```python
from build123d import *

# Parameters (mm, degrees)
SALIENTE_EXTRUIR1_DEPTH = 15
CROQUIS2_R              = 7
CORTAR_EXTRUIR1_DEPTH   = 135.246042772


with BuildPart() as part:
    # Croquis1 → Saliente-Extruir1 (new body)
    with BuildSketch(Plane.XY):
        with BuildLine():
            ThreePointArc((22.960111456, -43.287795993), (49, 0), (22.960111456, 43.287795993))
            ThreePointArc((22.960111456, 43.287795993), (17.471680778, 49.356927241), (17.149797537, 57.533333333))
            ThreePointArc((17.149797537, 57.533333333), (12.479188654, 75.97188693), (-6.126315717, 79.925373134))
            ThreePointArc((-6.126315717, 79.925373134), (-35.730309716, 61.63434209), (-55.523644659, 33.012983471))
            ThreePointArc((-55.523644659, 33.012983471), (-64.981782963, 22.905981014), (-78.737580645, 21.361342246))
            ThreePointArc((-78.737580645, 21.361342246), (-106, 0), (-78.737580645, -21.361342246))
            ThreePointArc((-78.737580645, -21.361342246), (-64.981782963, -22.905981014), (-55.523644659, -33.012983471))
            ThreePointArc((-55.523644659, -33.012983471), (-35.730309716, -61.63434209), (-6.126315717, -79.925373134))
            ThreePointArc((-6.126315717, -79.925373134), (12.479188654, -75.97188693), (17.149797537, -57.533333333))
            ThreePointArc((17.149797537, -57.533333333), (17.471680778, -49.356927241), (22.960111456, -43.287795993))
        make_face()
    extrude(amount=-SALIENTE_EXTRUIR1_DEPTH)

    # Croquis2 → Cortar-Extruir1 (cut, through all)
    with BuildSketch(Plane.XY):
        with Locations((0, 63)):
            Circle(CROQUIS2_R)
        with Locations((-84, 0)):
            Circle(CROQUIS2_R)
        with Locations((0, -63)):
            Circle(CROQUIS2_R)
        with BuildLine():
            Line((-2, 30.535898385), (-2, 26.925824036))
            ThreePointArc((-2, 26.925824036), (-6.988114218, 26.07999731), (-11.73086121, 24.318447633))
            Line((-11.73086121, 24.318447633), (-13.535898385, 27.444863729))
            ThreePointArc((-13.535898385, 27.444863729), (-19, 32.908965344), (-17, 25.444863729))
            Line((-17, 25.444863729), (-15.194962825, 22.318447633))
            ThreePointArc((-15.194962825, 22.318447633), (-19.091883092, 19.091883092), (-22.318447633, 15.194962825))
            Line((-22.318447633, 15.194962825), (-25.444863729, 17))
            ThreePointArc((-25.444863729, 17), (-32.908965344, 19), (-27.444863729, 13.535898385))
            Line((-27.444863729, 13.535898385), (-24.318447633, 11.73086121))
            ThreePointArc((-24.318447633, 11.73086121), (-26.07999731, 6.988114218), (-26.925824036, 2))
            Line((-26.925824036, 2), (-30.535898385, 2))
            ThreePointArc((-30.535898385, 2), (-38, 0), (-30.535898385, -2))
            Line((-30.535898385, -2), (-26.925824036, -2))
            ThreePointArc((-26.925824036, -2), (-26.07999731, -6.988114218), (-24.318447633, -11.73086121))
            Line((-24.318447633, -11.73086121), (-27.444863729, -13.535898385))
            ThreePointArc((-27.444863729, -13.535898385), (-32.908965344, -19), (-25.444863729, -17))
            Line((-25.444863729, -17), (-22.318447633, -15.194962825))
            ThreePointArc((-22.318447633, -15.194962825), (-19.091883092, -19.091883092), (-15.194962825, -22.318447633))
            Line((-15.194962825, -22.318447633), (-17, -25.444863729))
            ThreePointArc((-17, -25.444863729), (-19, -32.908965344), (-13.535898385, -27.444863729))
            Line((-13.535898385, -27.444863729), (-11.73086121, -24.318447633))
            ThreePointArc((-11.73086121, -24.318447633), (-6.988114218, -26.07999731), (-2, -26.925824036))
            Line((-2, -26.925824036), (-2, -30.535898385))
            ThreePointArc((-2, -30.535898385), (0, -38), (2, -30.535898385))
            Line((2, -30.535898385), (2, -26.925824036))
            ThreePointArc((2, -26.925824036), (6.988114218, -26.07999731), (11.73086121, -24.318447633))
            Line((11.73086121, -24.318447633), (13.535898385, -27.444863729))
            ThreePointArc((13.535898385, -27.444863729), (19, -32.908965344), (17, -25.444863729))
            Line((17, -25.444863729), (15.194962825, -22.318447633))
            ThreePointArc((15.194962825, -22.318447633), (19.091883092, -19.091883092), (22.318447633, -15.194962825))
            Line((22.318447633, -15.194962825), (25.444863729, -17))
            ThreePointArc((25.444863729, -17), (32.908965344, -19), (27.444863729, -13.535898385))
            Line((27.444863729, -13.535898385), (24.318447633, -11.73086121))
            ThreePointArc((24.318447633, -11.73086121), (26.07999731, -6.988114218), (26.925824036, -2))
            Line((26.925824036, -2), (30.535898385, -2))
            ThreePointArc((30.535898385, -2), (38, 0), (30.535898385, 2))
            Line((30.535898385, 2), (26.925824036, 2))
            ThreePointArc((26.925824036, 2), (26.07999731, 6.988114218), (24.318447633, 11.73086121))
            Line((24.318447633, 11.73086121), (27.444863729, 13.535898385))
            ThreePointArc((27.444863729, 13.535898385), (32.908965344, 19), (25.444863729, 17))
            Line((25.444863729, 17), (22.318447633, 15.194962825))
            ThreePointArc((22.318447633, 15.194962825), (19.091883092, 19.091883092), (15.194962825, 22.318447633))
            Line((15.194962825, 22.318447633), (17, 25.444863729))
            ThreePointArc((17, 25.444863729), (19, 32.908965344), (13.535898385, 27.444863729))
            Line((13.535898385, 27.444863729), (11.73086121, 24.318447633))
            ThreePointArc((11.73086121, 24.318447633), (6.988114218, 26.07999731), (2, 26.925824036))
            Line((2, 26.925824036), (2, 30.535898385))
            ThreePointArc((2, 30.535898385), (0, 38), (-2, 30.535898385))
        make_face()
    extrude(amount=-CORTAR_EXTRUIR1_DEPTH, mode=Mode.SUBTRACT)


solid = part.part
```
Work out the finished part from the listing and answer in its coordinate system (mm). A direction names the side the tool comes from. Round coordinates to 2 decimals unless told otherwise and drop trailing zeros. Write each loop counter-clockwise with the first axis right and the second up, starting at its lowest first coordinate (ties: lowest second). Pieces come first, ordered by that corner, then holes.
1) Flat-ended cylindrical pins translate along their axes: P1, Ø3, axis at y = 62.5, z = -12, coming from the +X side; P2, Ø9, axis at x = -17, y = 29.44, coming from the -Z side; P3, Ø1.8, axis at x = 29.5, z = -8.5, coming from the -Y side; P4, Ø6, axis at y = 10, z = -7, coming from the -X side. Find the tip coordinate at first contact, or state that the pin passes through.
2) A cutting plane is placed at D-D on z = -2.5. Give the number of separate pieces and of enclosed holes in the cut face, and give its area (3 significant figures).
3) A cutting plane is placed at A-A on y = 0. Determine the outline of the cut face in (x, z), and give its area (3 significant figures).
4) Consider probe 1 along Y at (x, z) = (0, -7.75); probe 2 along Y at (x, z) = (-5.5, -10.25); probe 3 along X at (y, z) = (24, -10.5). Determine where each line is inside the solid, lowest interval first.
5) Determine the mould class of faces 1 (the face through (-47, 1, -15)), 2 (the face through (17.516, 49.249, -7.395)), 3 (the face through (-19.042, 19.142, -7.395)) for opening direction X: pulls with the +X half, pulls with the -X half, needs draft (parallel to the pull), parting line crosses it, or undercut.
6) A cutting plane is placed at C-C on y = -63. Determine the outline of the cut face in (x, z), and give its area (3 significant figures).
7) A cutting plane is placed at B-B on x = -83.5. Determine the outline of the cut face in (y, z), and give its area (3 significant figures).
8) Which of the six approach directions +Z, -Z, +X, -X, +Y, -Y give full straight-line access (tool end or side, diameter ignored) to faces 4 (the face through (-64.8, 23, -7.4)), 5 (the face through (19.042, -19.142, -7.395))?
Entries:
1. P1: stops at x = 18
1. P2: stops at z = -15
1. P3: stops at y = -39.79
1. P4: stops at x = -104.86
2. separate pieces: 1
2. enclosed holes: 4
2. area: 10,600 mm2
3. outline: (-106, -15) - (-91, -15) - (-91, 0) - (-106, 0) - close; (-77, -15) - (-38, -15) - (-38, 0) - (-77, 0) - close; (38, -15) - (49, -15) - (49, 0) - (38, 0) - close
3. area: 975 mm2
4. probe 1: y = -81 to -70, -56 to -38, 38 to 56, 70 to 81
4. probe 2: y = -80.14 to -67.33, -58.67 to -26.43, 26.43 to 58.67, 67.33 to 80.14
4. probe 3: x = -63.07 to -16.17, 16.17 to 42.72
5. face 1: needs draft
5. face 2: pulls with the +X half
5. face 3: undercut
6. outline: (-34.26, -15) - (-7, -15) - (-7, 0) - (-34.26, 0) - close; (7, -15) - (18, -15) - (18, 0) - (7, 0) - close
6. area: 574 mm2
7. outline: (-21.99, -15) - (-6.98, -15) - (-6.98, 0) - (-21.99, 0) - close; (6.98, -15) - (21.99, -15) - (21.99, 0) - (6.98, 0) - close
7. area: 450 mm2
8. face 4: +Z, -Z, +Y
8. face 5: +Z, -Z
